from build123d import *

# Parameters (mm, degrees)
MODEL_R             = 11.05
MODEL_R_2           = 22.5
MODEL_R_3           = 3
MODEL_R_4           = 3.5
MODEL_R_5           = 2
MODEL_W             = 5.4
MODEL_H             = 15.4
MODEL_W_2           = 5
MODEL_H_2           = 15
MODEL_W_3           = 15.4
MODEL_H_3           = 5.4
BOSS_EXTRUDE1_DEPTH = 17


with BuildPart() as part:
    # Model → Boss-Extrude1 (new body)
    with BuildSketch(Plane.XY):
        with BuildLine():
            Line((170.621850122, -313.319218198), (170.621850122, -293.319218198))
            Line((170.621850122, -293.319218198), (175.821850122, -293.319218198))
            Line((175.821850122, -293.319218198), (175.821850122, -273.319218198))
            Line((175.821850122, -273.319218198), (170.621850122, -273.319218198))
            Line((170.621850122, -273.319218198), (170.621850122, -253.319218198))
            Line((170.621850122, -253.319218198), (175.821850122, -253.319218198))
            Line((175.821850122, -253.319218198), (175.821850122, -233.319218198))
            Line((175.821850122, -233.319218198), (170.621850122, -233.319218198))
            Line((170.621850122, -233.319218198), (170.621850122, -208.319218198))
            Line((170.621850122, -208.319218198), (175.821850122, -208.319218198))
            Line((175.821850122, -208.319218198), (175.821850122, -188.319218198))
            ThreePointArc((175.821850122, -188.319218198), (164.106121369, -160.034946951), (135.821850122, -148.319218198))
            Line((135.821850122, -148.319218198), (-124.178149879, -148.319218198))
            ThreePointArc((-124.178149879, -148.319218198), (-152.462421126, -160.034946951), (-164.178149878, -188.319218198))
            Line((-164.178149878, -188.319218198), (-164.178149878, -488.469218198))
            Line((-164.178149878, -488.469218198), (-126.678149879, -488.469218198))
            Line((-126.678149879, -488.469218198), (-126.678149879, -483.269218198))
            Line((-126.678149879, -483.269218198), (-96.678149879, -483.269218198))
            Line((-96.678149879, -483.269218198), (-96.678149879, -488.469218198))
            Line((-96.678149879, -488.469218198), (-66.678149879, -488.469218198))
            Line((-66.678149879, -488.469218198), (-66.678149879, -483.269218198))
            Line((-66.678149879, -483.269218198), (23.321850122, -483.269218198))
            Line((23.321850122, -483.269218198), (23.321850122, -488.469218198))
            Line((23.321850122, -488.469218198), (53.321850122, -488.469218198))
            Line((53.321850122, -488.469218198), (53.321850122, -483.269218198))
            Line((53.321850122, -483.269218198), (83.321850122, -483.269218198))
            Line((83.321850122, -483.269218198), (83.321850122, -488.469218198))
            Line((83.321850122, -488.469218198), (113.321850122, -488.469218198))
            Line((113.321850122, -488.469218198), (113.321850122, -483.269218198))
            Line((113.321850122, -483.269218198), (143.321850122, -483.269218198))
            Line((143.321850122, -483.269218198), (143.321850122, -488.469218198))
            Line((143.321850122, -488.469218198), (158.321850122, -488.469218198))
            Line((158.321850122, -488.469218198), (158.321850122, -483.469218198))
            Line((158.321850122, -483.469218198), (170.821850122, -470.969218198))
            Line((170.821850122, -470.969218198), (175.821850122, -470.969218198))
            Line((175.821850122, -470.969218198), (175.821850122, -455.969218198))
            Line((175.821850122, -455.969218198), (170.621850122, -455.969218198))
            Line((170.621850122, -455.969218198), (170.621850122, -425.769218198))
            Line((170.621850122, -425.769218198), (175.821850122, -425.769218198))
            Line((175.821850122, -425.769218198), (175.821850122, -358.519218198))
            Line((175.821850122, -358.519218198), (170.621850122, -358.519218198))
            Line((170.621850122, -358.519218198), (170.621850122, -338.319218198))
            Line((170.621850122, -338.319218198), (175.821850122, -338.319218198))
            Line((175.821850122, -338.319218198), (175.821850122, -313.319218198))
            Line((175.821850122, -313.319218198), (170.621850122, -313.319218198))
        make_face()
        with Locations((-75.178149879, -219.469218198)):
            Circle(MODEL_R, mode=Mode.SUBTRACT)
        with Locations((150.821850122, -425.469218198)):
            Circle(MODEL_R, mode=Mode.SUBTRACT)
        with Locations((-5.678149878, -219.469218198)):
            Circle(MODEL_R_2, mode=Mode.SUBTRACT)
        with Locations((13.821850122, -253.244208946)):
            Circle(MODEL_R_3, mode=Mode.SUBTRACT)
        with Locations((13.821850122, -185.69422745)):
            Circle(MODEL_R_3, mode=Mode.SUBTRACT)
        with Locations((-52.178149879, -219.469218198)):
            Circle(MODEL_R_3, mode=Mode.SUBTRACT)
        with Locations((150.821850122, -240.469218198)):
            Circle(MODEL_R_4, mode=Mode.SUBTRACT)
        with Locations((150.821850122, -225.469218198)):
            Circle(MODEL_R_4, mode=Mode.SUBTRACT)
        with Locations((106.671850121, -337.269218198)):
            Circle(MODEL_R_5, mode=Mode.SUBTRACT)
        with Locations((145.471850121, -260.469218198)):
            Circle(MODEL_R_5, mode=Mode.SUBTRACT)
        with Locations((145.471850121, -337.269218198)):
            Circle(MODEL_R_5, mode=Mode.SUBTRACT)
        with Locations((106.671850121, -260.469218198)):
            Circle(MODEL_R_5, mode=Mode.SUBTRACT)
        with BuildLine():
            Line((-49.178149879, -373.469218198), (-49.178149878, -423.469218198))
            ThreePointArc((-49.178149878, -423.469218198), (5.821850122, -478.469218198), (60.821850122, -423.469218198))
            Line((60.821850122, -423.469218198), (60.821850122, -373.469218198))
            ThreePointArc((60.821850122, -373.469218198), (49.106121369, -345.184946951), (20.821850122, -333.469218198))
            Line((20.821850122, -333.469218198), (-9.178149878, -333.469218198))
            ThreePointArc((-9.178149878, -333.469218198), (-37.462421126, -345.184946951), (-49.178149879, -373.469218198))
        make_face(mode=Mode.SUBTRACT)
        with Locations((-5.678149879, -167.819218198)):
            Rectangle(MODEL_W, MODEL_H, mode=Mode.SUBTRACT)
        with Locations((-5.678149879, -271.119218198)):
            Rectangle(MODEL_W, MODEL_H, mode=Mode.SUBTRACT)
        with Locations((73.321850122, -462.969218198)):
            Rectangle(MODEL_W_2, MODEL_H_2, mode=Mode.SUBTRACT)
        with Locations((148.321850122, -210.819218198)):
            Rectangle(MODEL_W_3, MODEL_H_3, mode=Mode.SUBTRACT)
        with Locations((148.321850122, -355.819218198)):
            Rectangle(MODEL_W_3, MODEL_H_3, mode=Mode.SUBTRACT)
        with Locations((-156.678149878, -450.969218198)):
            Rectangle(MODEL_W_2, MODEL_H_2, mode=Mode.SUBTRACT)
        with Locations((-61.678149878, -462.969218198)):
            Rectangle(MODEL_W_2, MODEL_H_2, mode=Mode.SUBTRACT)
    extrude(amount=BOSS_EXTRUDE1_DEPTH)


solid = part.part
The listing builds one solid part. Answer for the finished solid, in the listing's coordinates (mm). A direction names the side the tool comes from. Coordinates: 2 decimals unless noted, no trailing zeros. Loops run counter-clockwise (first coordinate to the right, second up) from the corner with the lowest first, then second, coordinate; pieces in that order, holes last.
1) A tool of negligible diameter and unlimited length cuts with its end or side. For faces 1 (the face through (148, -213.519, 8)), 2 (the face through (-22, -483.269, 8)), 3 (the face through (170.622, -441, 8)), from which of +Z, -Z, +X, -X, +Y, -Y can it reach the whole face along a straight path? Write none if from no direction.
2) Determine the mould class of faces 4 (the face through (-8.378, -168, 8)), 5 (the face through (-82, -488.469, 8)), 6 (the face through (175.822, -283, 8)) for opening direction Y: pulls with the +Y half, pulls with the -Y half, needs draft (parallel to the pull), parting line crosses it, or undercut.
3) Find section C-C on z = 8. Give the number of separate pieces and of enclosed holes in the cut face, then the cut area to 3 significant figures.
4) Find the intervals of material crossed by L1, parallel to X at y = -405, z = 7.75; L2, parallel to X at y = -223, z = 5.5; L3, parallel to X at y = -424, z = 3.5, in increasing order.
5) Find section A-A on y = -389. Write down the section's boundary in (x, z).
6) Flat-ended cylindrical pins translate along their axes: pin 1 Ø5.5 at (x, z) = (-62.5, 10.5) entering from -Y; pin 2 Ø3 at (y, z) = (-231.5, 13.5) entering from +X; pin 3 Ø5.5 at (x, z) = (173.5, 6.5) entering from +Y (3 decimals). Find the tip coordinate at first contact, or state that the pin passes through.
7) Find section B-B on x = -35.5. Write down the section's boundary in (y, z).
Values:
1. face 1: +Z, -Z
1. face 2: +Z, -Z, -Y
1. face 3: +Z, -Z, +X
2. face 4: undercut
2. face 5: pulls with the -Y half
2. face 6: needs draft
3. separate pieces: 1
3. enclosed holes: 20
3. area: 96,100 mm2
4. L1: x = -164.18 to -49.18, 60.82 to 175.82
4. L2: x = -164.18 to -85.65, -64.71 to -27.9, 16.54 to 148.34, 153.3 to 170.62
4. L3: x = -164.18 to -49.18, 60.82 to 139.87, 161.77 to 175.82
5. outline: (-164.18, 0) - (-49.18, 0) - (-49.18, 17) - (-164.18, 17) - close; (60.82, 0) - (175.82, 0) - (175.82, 17) - (60.82, 17) - close
6. pin 1: stops at y = -483.27
6. pin 2: stops at x = 170.62
6. pin 3: stops at y = -168.825
7. outline: (-483.27, 0) - (-459.77, 0) - (-459.77, 17) - (-483.27, 17) - close; (-343.35, 0) - (-148.32, 0) - (-148.32, 17) - (-343.35, 17) - close
